The listing builds one solid part. Answer for the finished solid, in the listing's coordinates (mm). A direction names the side the tool comes from. Round coordinates to 2 decimals unless told otherwise and drop trailing zeros. Write each loop counter-clockwise with the first axis right and the second up, starting at its lowest first coordinate (ties: lowest second). Pieces come first, ordered by that corner, then holes. Notation, with made-up numbers: (81, -26) - (137, -26) arc R24 ccw to (137, 10) - close; hole circle Ø3 at (-2, -17.5). An arc over 180 degrees is marked (long way). Return JSON: item names as keys, results as strings. Group by question number.
(1) Section B-B, the plane z = 25.5 is taken. Write down the section's boundary in (x, y), then the cut area to 3 significant figures.
(2) Each of these flat-tipped pins is pushed along its axis until it touches: pin 1 (3 mm diameter, centred on x = 3.35, z = 46.86, fed in from +Y); pin 2 (5 mm diameter, centred on x = -0.15, z = -31.43, fed in from +Y). Where does it stop, or does it pass through?
(3) Find the intervals of material crossed by line 1 along X through (y, z) = (-0.6, -31.5); line 2 along X through (y, z) = (-0.45, -15); line 3 along X through (y, z) = (-0.05, 38), in increasing order. Write a range as [from, to].
(4) Determine the mould class of faces 1 (the cylindrical face through (-0.36, -0.49, -29.81)), 2 (the flat face through (4, 0, -9)) for opening direction X: +X half, -X half, draft (parallel to the pull), parting line (faces both ways), or undercut.
(5) Which of the six approach directions +Z, -Z, +X, -X, +Y, -Y give full straight-line access (tool end or side, diameter ignored) to faces 3 (the flat face through (-0.22, -0.49, -13.51)), 4 (the flat face through (4, -1, -9))?
(6) Section A-A, the plane y = -0.2 is taken. Give the number of separate pieces and of enclosed holes in the cut face, then the cut area to 3 significant figures.
```python
from build123d import *

# Parameters (mm, degrees)
F0_W     = 14
F0_H     = 100
F0_R     = 1.64
F1_DEPTH = 1


with BuildPart() as f1:
    # F0 (on Front) → F1 (new body)
    with BuildSketch(Plane.XZ):
        with Locations((-0.146341, 1.690268)):
            Rectangle(F0_W, F0_H)
        with Locations((-0.146341, -44.184732)):
            Circle(F0_R, mode=Mode.SUBTRACT)
        with Locations((-0.146341, -31.434732)):
            Circle(F0_R, mode=Mode.SUBTRACT)
        Polygon((-5.146341, -19.405732), (4.853659, -27.309732), (-5.146341, -27.309732), align=None, mode=Mode.SUBTRACT)
        Polygon((-5.146341, -17.405732), (4.853659, -9.501732), (4.853659, -25.309732), align=None, mode=Mode.SUBTRACT)
        Polygon((-5.146341, -15.405732), (-5.146341, 0.402268), (4.853659, -7.501732), align=None, mode=Mode.SUBTRACT)
        Polygon((4.853659, -5.499732), (-5.146341, 2.404268), (4.853659, 10.308268), align=None, mode=Mode.SUBTRACT)
        Polygon((-5.146341, 20.212268), (4.853659, 12.308268), (-5.146341, 4.404268), align=None, mode=Mode.SUBTRACT)
        Polygon((-5.146341, 22.214268), (4.853659, 30.118268), (4.853659, 14.310268), align=None, mode=Mode.SUBTRACT)
        Polygon((4.853659, 32.118268), (-5.146341, 24.214268), (-5.146341, 40.022268), align=None, mode=Mode.SUBTRACT)
        Polygon((-5.146341, 42.024268), (4.853659, 42.024268), (4.853659, 34.120268), align=None, mode=Mode.SUBTRACT)
        with Locations((-3.646341, 46.857268)):
            Circle(F0_R, mode=Mode.SUBTRACT)
        with Locations((3.353659, 46.857268)):
            Circle(F0_R, mode=Mode.SUBTRACT)
    extrude(amount=F1_DEPTH)


solid = f1.part
```
Working result:
{
 "1": {"outline": "(-7.15, -1) - (-5.15, -1) - (-5.15, 0) - (-7.15, 0) - close; (-3.52, -1) - (-0.99, -1) - (-0.99, 0) - (-3.52, 0) - close; (4.85, -1) - (6.85, -1) - (6.85, 0) - (4.85, 0) - close", "area": "6.53 mm^2"},
 "2": {"pin 1": "passes through", "pin 2": "stops at y = 0"},
 "3": {"line 1": "x = [-7.15, -1.79], [1.49, 6.85]", "line 2": "x = [-7.15, -5.15], [-4.63, -2.1], [4.85, 6.85]", "line 3": "x = [-7.15, -5.15], [-2.59, -0.05], [4.85, 6.85]"},
 "4": {"face 1": "undercut", "face 2": "draft"},
 "5": {"face 3": "+Y, -Y", "face 4": "+Z, -Z, +X, -X, -Y"},
 "6": {"separate pieces": "1", "enclosed holes": "12", "area": "813 mm^2"}
}
